Can you work these out from the model? Positions are in its coordinate system, mm. Round coordinates to 2 decimals unless told otherwise and drop trailing zeros. Loops run counter-clockwise (first coordinate to the right, second up) from the corner with the lowest first, then second, coordinate; pieces in that order, holes last.
```python
from build123d import *

# Parameters (mm, degrees)
SKICA1_W                 = 170
SKICA1_H                 = 25
P_IDAT_VYSUNUT_M1_DEPTH  = 3
SKICA2_W                 = 3
SKICA2_H                 = 5
ODEBRAT_VYSUNUT_M2_DEPTH = 86.966563267
SKICA3_R                 = 2
ODEBRAT_VYSUNUT_M3_DEPTH = 86.966563267


with BuildPart() as part:
    # Skica1 → Přidat vysunutím1 (new body)
    with BuildSketch(Plane(origin=(0, 0, 0), x_dir=(1, 0, 0), z_dir=(0, 1, 0))):
        Rectangle(SKICA1_W, SKICA1_H)
    extrude(amount=P_IDAT_VYSUNUT_M1_DEPTH)

    # Skica2 → Odebrat vysunutím2 (cut, through all)
    with BuildSketch(Plane(origin=(0, 0, 0), x_dir=(1, 0, 0), z_dir=(0, 1, 0))):
        with Locations((0, 5)):
            Rectangle(SKICA2_W, SKICA2_H)
        with Locations((0, -5)):
            Rectangle(SKICA2_W, SKICA2_H)
        with Locations((-66.5, 5)):
            Rectangle(SKICA2_W, SKICA2_H)
        with Locations((-66.5, -5)):
            Rectangle(SKICA2_W, SKICA2_H)
        with Locations((66.5, 7)):
            Rectangle(SKICA2_W, SKICA2_H)
        with Locations((66.5, -3)):
            Rectangle(SKICA2_W, SKICA2_H)
    extrude(amount=ODEBRAT_VYSUNUT_M2_DEPTH, mode=Mode.SUBTRACT)

    # Skica3 → Odebrat vysunutím3 (cut, through all)
    with BuildSketch(Plane(origin=(0, 0, 0), x_dir=(1, 0, 0), z_dir=(0, 1, 0))):
        with Locations(Location((-78.65, 0.29, 0), (0, 0, 270))):
            Circle(SKICA3_R)
        with Locations(Location((78.83, 0.29, 0), (0, 0, 270))):
            Circle(SKICA3_R)
    extrude(amount=ODEBRAT_VYSUNUT_M3_DEPTH, mode=Mode.SUBTRACT)


solid = part.part
```
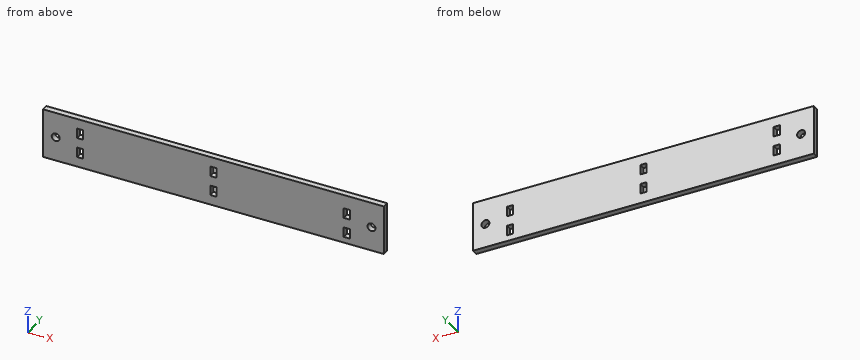
(1) Suppose I cut it at A-A (x = 78.83). Write out the boundary of the cut face in (y, z).
(2) If I drill on line 1 (X direction, y = 0.9, z = 7); line 2 (X direction, y = 2.15, z = 3.75); line 3 (X direction, y = 0.75, z = -0.29), over which ranges is the centre line in solid material (lowest first)?
(3) Suppose I cut it at B-B (z = 4). Write out the boundary of the cut face in (x, y), then the cut area to 3 significant figures.
Check result:
1. outline: (0, -12.5) - (3, -12.5) - (3, -2.29) - (0, -2.29) - close; (0, 1.71) - (3, 1.71) - (3, 12.5) - (0, 12.5) - close
2. line 1: x = -85 to -68, -65 to -1.5, 1.5 to 85
2. line 2: x = -85 to -68, -65 to -1.5, 1.5 to 65, 68 to 85
2. line 3: x = -85 to -80.65, -76.65 to 76.83, 80.83 to 85
3. outline: (-85, 0) - (-68, 0) - (-68, 3) - (-85, 3) - close; (-65, 0) - (-1.5, 0) - (-1.5, 3) - (-65, 3) - close; (1.5, 0) - (65, 0) - (65, 3) - (1.5, 3) - close; (68, 0) - (85, 0) - (85, 3) - (68, 3) - close
3. area: 483 mm2
